```python
from build123d import *

# Parameters (mm, degrees)
SKETCH1_R           = 11
BOSS_EXTRUDE1_DEPTH = 2
SKETCH2_R           = 8.5
SKETCH2_R_2         = 7.5
BOSS_EXTRUDE2_DEPTH = 6
SKETCH3_R           = 2.6
CUT_EXTRUDE1_DEPTH  = 17.673332001
SKETCH4_R           = 7.43362206
BOSS_EXTRUDE3_DEPTH = 4.5
FILLET1_R           = 3
FILLET2_R           = 1
FILLET3_R           = 0.5


with BuildPart() as part:
    # Sketch1 → Boss-Extrude1 (new body)
    with BuildSketch(Plane(origin=(0, 0, 0), x_dir=(1, 0, 0), z_dir=(0, 1, 0))):
        with Locations(Location((0, 0, 0), (0, 0, 270))):
            Circle(SKETCH1_R)
    extrude(amount=BOSS_EXTRUDE1_DEPTH)

    # Sketch2 → Boss-Extrude2 (add)
    with BuildSketch(Plane(origin=(0, 2, 0), x_dir=(1, 0, 0), z_dir=(0, 1, 0))):
        with Locations(Location((0, 0, 0), (0, 0, 270))):
            Circle(SKETCH2_R)
        with Locations(Location((0, 0, 0), (0, 0, 270))):
            Circle(SKETCH2_R_2, mode=Mode.SUBTRACT)
    extrude(amount=BOSS_EXTRUDE2_DEPTH)

    # Sketch3 → Cut-Extrude1 (cut, through all)
    with BuildSketch(Plane(origin=(0, 2, 0), x_dir=(1, 0, 0), z_dir=(0, 1, 0))):
        with Locations(Location((0, 0, 0), (0, 0, 270))):
            Circle(SKETCH3_R)
    extrude(amount=-CUT_EXTRUDE1_DEPTH, mode=Mode.SUBTRACT)

    # Sketch4 → Boss-Extrude3 (add)
    with BuildSketch(Plane.XZ):
        with Locations(Location((0, 0, 0), (0, 0, 270))):
            Circle(SKETCH4_R)
        Polygon((0, -5.311622477), (4.6, -2.655811238), (4.6, 2.655811238), (0, 5.311622477), (-4.6, 2.655811238), (-4.6, -2.655811238), align=None, mode=Mode.SUBTRACT)
    extrude(amount=BOSS_EXTRUDE3_DEPTH)

    # Fillet1
    fillet1_edges = [part.edges().sort_by_distance(p)[0] for p in [
        (0, 0, 7.43362206),
    ]]
    fillet(fillet1_edges, radius=FILLET1_R)

    # Fillet2
    fillet2_edges = [part.edges().sort_by_distance(p)[0] for p in [
        (0, -4.5, 7.43362206),
    ]]
    fillet(fillet2_edges, radius=FILLET2_R)

    # Fillet3
    fillet3_edges = [part.edges().sort_by_distance(p)[0] for p in [
        (0, 8, -8.5),
        (0, 8, -7.5),
    ]]
    fillet(fillet3_edges, radius=FILLET3_R - 0.0001)  # a hair under: the kernel refuses the full size


solid = part.part
```
Geometry: final body of the model. Coordinates: model frame, mm. A direction names the side the tool comes from. Round coordinates to 2 decimals unless told otherwise and drop trailing zeros. Write each loop counter-clockwise with the first axis right and the second up, starting at its lowest first coordinate (ties: lowest second). Pieces come first, ordered by that corner, then holes. Notation, with made-up numbers: M -0.5,-30 L 12.5,-30 A21 ccw 12.5,-9 Z; hole C 67.25,88.5 d5. An arc over 180 degrees is marked long. Answer in a Markdown table with one row per item. Add a question column.
(1) Cut plane C-C, the plane y = 5.25. Return the cut outline in (x, z).
(2) Reachability of faces 1 (the face through (0.78, 1.01, 2.48)), 2 (the face through (-4.52, -3.25, 5.9)), 3 (the face through (0.33, 4.712, -7.493)) from +Z, -Z, +X, -X, +Y, -Y: full face, straight path, thin tool, end or side. Return the list, or none.
(3) Cut plane B-B, the plane y = -0.75. Return the cut outline in (x, z), then the cut area to 3 significant figures.
(4) Draft query along X for faces 4 (the face through (8.428, 4.712, -1.107)), 5 (the face through (-5, -4.5, 0)), 6 (the face through (2, 0, 2)). Return one class per face: pulls with the +X half, pulls with the -X half, needs draft (parallel to the pull), parting line crosses it, or undercut.
(5) Contact query for flat-ended pins moving along their axis: pin 1 (1 mm diameter, centred on x = 3.5, y = 4.5, fed in from -Z); pin 2 (4 mm diameter, centred on y = 1, z = 8.5, fed in from +X); pin 3 (2 mm diameter, centred on x = -1, y = -3, fed in from -Z). Output: stop coordinate, or through.
(6) Ray query, L1, parallel to X at y = 0.75, z = 0; L2, parallel to X at y = 5.4, z = 0; L3, parallel to Z at x = -2.5, y = 5.75. Return the intervals inside material, ascending.
Established:
| question | item | result |
|---|---|---|
| 1 | outline | C 0,0 d17; hole C 0,0 d15 |
| 2 | face 1 | +Y, -Y |
| 2 | face 2 | -Y |
| 2 | face 3 | +Y |
| 3 | outline | C 0,0 d16.9; hole M -4.6,-2.66 L 0,-5.31 L 4.6,-2.66 L 4.6,2.66 L 0,5.31 L -4.6,2.66 Z |
| 3 | area | 151 mm² |
| 4 | face 4 | parting line crosses it |
| 4 | face 5 | needs draft |
| 4 | face 6 | undercut |
| 5 | pin 1 | z = -7.95 |
| 5 | pin 2 | x = 8.87 |
| 5 | pin 3 | z = -7.56 |
| 6 | L1 | -11 to -2.6, 2.6 to 11 |
| 6 | L2 | -8.5 to -7.5, 7.5 to 8.5 |
| 6 | L3 | -8.12 to -7.07, 7.07 to 8.12 |
